Part model, mm, in its own coordinate system. A direction names the side the tool comes from. Round coordinates to 2 decimals unless told otherwise and drop trailing zeros. Loops run counter-clockwise (first coordinate to the right, second up) from the corner with the lowest first, then second, coordinate; pieces in that order, holes last.
from build123d import *

# Parameters (mm, degrees)
SKETCH1_W           = 12
SKETCH1_H           = 12
BOSS_EXTRUDE1_DEPTH = 2
SKETCH3_W           = 12
SKETCH3_H           = 2
BOSS_EXTRUDE2_DEPTH = 5
CUT_EXTRUDE1_DEPTH  = 5
SKETCH5_R           = 1.6
CUT_EXTRUDE2_DEPTH  = 5
SKETCH7_R           = 1.25
CUT_EXTRUDE3_DEPTH  = 5
BOSS_EXTRUDE4_DEPTH = 1.5


with BuildPart() as part:
    # Sketch1 → Boss-Extrude1 (new body)
    with BuildSketch(Plane(origin=(0, 0, 0), x_dir=(0, 0, -1), z_dir=(1, 0, 0))):
        with Locations((0, -1.5)):
            Rectangle(SKETCH1_W, SKETCH1_H)
    extrude(amount=BOSS_EXTRUDE1_DEPTH)

    # Sketch3 → Boss-Extrude2 (add)
    with BuildSketch(Plane.ZY):
        with Locations((0, 3.5)):
            Rectangle(SKETCH3_W, SKETCH3_H)
    extrude(amount=BOSS_EXTRUDE2_DEPTH)

    # Sketch4 → Cut-Extrude1 (cut)
    with BuildSketch(Plane(origin=(2, 0, 0), x_dir=(0, 0, -1), z_dir=(1, 0, 0))):
        Polygon((-6, -2.5), (-1, -7.5), (-6, -7.5), align=None)
        Polygon((1, -7.5), (6, -7.5), (6, -2.5), align=None)
    extrude(amount=-CUT_EXTRUDE1_DEPTH, mode=Mode.SUBTRACT)

    # Sketch5 → Cut-Extrude2 (cut)
    with BuildSketch(Plane(origin=(2, 0, 0), x_dir=(0, 0, -1), z_dir=(1, 0, 0))):
        with Locations((0, -1.511770417)):
            Circle(SKETCH5_R)
    extrude(amount=-CUT_EXTRUDE2_DEPTH, mode=Mode.SUBTRACT)

    # Sketch7 → Cut-Extrude3 (cut)
    with BuildSketch(Plane.XZ.offset(-2.5)):
        with Locations((-2.5, 3)):
            Circle(SKETCH7_R)
        with Locations((-2.5, -3)):
            Circle(SKETCH7_R)
    extrude(amount=-CUT_EXTRUDE3_DEPTH, mode=Mode.SUBTRACT)

    # Sketch8 → Boss-Extrude4 (add)
    with BuildSketch(Plane.XY.offset(6)):
        Polygon((-5, 2.5), (0, 2.5), (0, -2.5), align=None)
    boss_extrude4 = extrude(amount=-BOSS_EXTRUDE4_DEPTH)

    # Mirror1: Boss-Extrude4 across plane
    add(boss_extrude4.mirror(Plane.XY))


solid = part.part
1) Tool access for faces 5 (the face through (0, -4, 0)), 6 (the face through (1, -5, -3.5)): list every direction of +Z, -Z, +X, -X, +Y, -Y with a clear straight run to the whole face (end or side of a thin tool).
Values:
face 5: -X, -Y
face 6: -Z, +X, -X, -Y
2) Mould opens along Z. For faces 1 (the face through (-1.31, 3.49, 3.38)), 2 (the face through (-1, 2, -6)), 3 (the face through (-2.5, 0, -5.3)), 4 (the face through (-2, 2.5, 0)) say: released by +Z, released by -Z, zero draft, split by the parting line, or undercut.
Values:
face 1: undercut
face 2: released by -Z
face 3: zero draft
face 4: undercut
3) Drop flat-ended pins along their axis: pin 1 Ø3 at (y, z) = (-1.51, 0) entering from -X; pin 2 Ø3 at (y, z) = (-0.5, -1) entering from -X; pin 3 Ø2 at (x, z) = (0.5, -3.5) entering from -Y. Give the stop position or say it passes through.
Values:
pin 1: passes through
pin 2: stops at x = 0
pin 3: stops at y = -6
4) Slice it at B-B, the plane x = -4. Give the cut face in (y, z), then the cut area to 3 significant figures.
Values:
outline: (1.5, -6) - (4.5, -6) - (4.5, 6) - (1.5, 6) - (1.5, 4.5) - (2.5, 4.5) - (2.5, -4.5) - (1.5, -4.5) - close
area: 27.0 mm2
5) Slice it at D-D, the plane x = -2.5. Give the cut face in (y, z), then the cut area to 3 significant figures.
Values:
outline: (0, -6) - (4.5, -6) - (4.5, -4.25) - (2.5, -4.25) - (2.5, -4.5) - (0, -4.5) - close; (0, 4.5) - (2.5, 4.5) - (2.5, 4.25) - (4.5, 4.25) - (4.5, 6) - (0, 6) - close; (2.5, -1.75) - (4.5, -1.75) - (4.5, 1.75) - (2.5, 1.75) - close
area: 21.5 mm2
6) Slice it at A-A, the plane z = 0. Give the cut face in (x, y).
Values:
outline: (-5, 2.5) - (0, 2.5) - (0, 0.09) - (2, 0.09) - (2, 4.5) - (-5, 4.5) - close; (0, -7.5) - (2, -7.5) - (2, -3.11) - (0, -3.11) - close
7) Wall check: line 1 along Z through (x, y) = (-2.5, 3.1); line 2 along X through (y, z) = (-4, 0.25); line 3 along Y through (x, z) = (-1.5, -5.5). Give the ranges that are in metal, low to high.
Values:
line 1: z = -6 to -4.25, -1.75 to 1.75, 4.25 to 6
line 2: x = 0 to 2
line 3: y = -1 to 4.5
8) Slice it at C-C, the plane y = -1.25. Give the cut face in (x, z), then the cut area to 3 significant figures.
Values:
outline: (-1.25, -6) - (2, -6) - (2, -1.58) - (0, -1.58) - (0, -4.5) - (-1.25, -4.5) - close; (-1.25, 4.5) - (0, 4.5) - (0, 1.58) - (2, 1.58) - (2, 6) - (-1.25, 6) - close
area: 21.4 mm2
